Model file for the job. Use its own axes, mm. A direction names the side the tool comes from. Give positions to 0.01 mm unless a question says otherwise; leave off trailing zeros. Order: outer loops, then holes, each group sorted by start corner. A loop starts at its lowest first (then second) coordinate and runs counter-clockwise, first axis right, second up. Notation, with made-up numbers: (38, 7) - (92, 7) arc R8 cw to (92, 18) - close; hole circle Ø9 at (42, 70.5). An arc over 180 degrees is marked (long way). Use CSV: the item, a comma, the result in double quotes. Start each with the question number.
(1) Band-saw the part on A-A, the plane z = -0.7. Give the cut face in (x, y), then the cut area to 3 significant figures.
(2) Pull direction X, two halves, no side cores. Call faces 3 (the flat face through (15, -1, -1)), 4 (the cylindrical face through (-4.524, -1.065, -0.219)), 5 (the flat face through (-15, -1, 40.5)), 6 (the flat face through (-15, -1, -7)): +X half, -X half, draft (parallel to the pull), parting line (faces both ways), or undercut.
(3) Band-saw the part on B-B, the plane x = -6.05. Give the cut face in (y, z).
(4) Tool access for faces 1 (the flat face through (-30, -1, 27.65)), 2 (the cylindrical face through (7.452, -1.065, 13.019)): list every direction of +Z, -Z, +X, -X, +Y, -Y with a clear straight run to the whole face (end or side of a thin tool).
(5) Band-saw the part on C-C, the plane y = -0.95. Count the separate pieces of the cut face and the enclosed holes in it, then the cut area to 3 significant figures.
(6) Probe L1, parallel to Z at x = -42, y = -1.3 (3 decimals); L2, parallel to Z at x = 9, y = -1.2; L3, parallel to X at y = -1.55, z = 35.5. List the from-to ranges inside material, lowest first.
(7) Drop a flat-ended pin along its axis: pin 1 Ø1.9 at (x, z) = (6.05, -0.7) entering from -Y. Give the stop position or say it passes through.
(8) Band-saw the part on D-D, the plane z = 11.6. Give the cut face in (x, y).
from build123d import *

# Parameters (mm, degrees)
F0_W     = 30
F0_H     = 81
F1_DEPTH = 2.1
F2_R     = 2.1
F2_R_2   = 1.6
F3_DEPTH = 2.101
F4_W     = 2.1
F4_H     = 12.85
F5_DEPTH = 30
F6_R     = 1.1
F7_DEPTH = 25


with BuildPart() as f1:
    # F0 (on Front) → F1 (new body)
    with BuildSketch(Plane.XZ):
        Rectangle(F0_W, F0_H)
    extrude(amount=F1_DEPTH)

    # F2 (on face) → F3 (cut, through all)
    with BuildSketch(Plane.XZ.offset(2.1)):
        with Locations((9, 35.6)):
            Circle(F2_R)
        with Locations((9, 11.6)):
            Circle(F2_R)
        with Locations((-9, 35.6)):
            Circle(F2_R)
        with Locations((-9, 11.6)):
            Circle(F2_R)
        with Locations((9, -9.2)):
            Circle(F2_R)
        with Locations((-9, -9.2)):
            Circle(F2_R)
        with Locations((6.05, -0.7)):
            Circle(F2_R_2)
        with Locations((-6.05, -0.7)):
            Circle(F2_R_2)
    extrude(amount=-F3_DEPTH, mode=Mode.SUBTRACT)

    # F4 (on face) → F5 (join)
    with BuildSketch(Plane(origin=(-15, 0, 0), x_dir=(0, -1, 0), z_dir=(-1, 0, 0))):
        with Locations((1.05, 34.075)):
            Rectangle(F4_W, F4_H)
    extrude(amount=F5_DEPTH)

    # F6 (on face) → F7 (cut)
    with BuildSketch(Plane.XZ.offset(2.1)):
        with Locations((-42, 38.175)):
            Circle(F6_R)
        with Locations((-42, 29.975)):
            Circle(F6_R)
    extrude(amount=-F7_DEPTH, mode=Mode.SUBTRACT)


solid = f1.part
Answer block:
1,outline,"(-15, -2.1) - (-7.65, -2.1) - (-7.65, 0) - (-15, 0) - close; (-4.45, -2.1) - (4.45, -2.1) - (4.45, 0) - (-4.45, 0) - close; (7.65, -2.1) - (15, -2.1) - (15, 0) - (7.65, 0) - close"
1,area,"49.6 mm2"
2,face 3,"+X half"
2,face 4,"undercut"
2,face 5,"draft"
2,face 6,"-X half"
3,outline,"(-2.1, -40.5) - (0, -40.5) - (0, -2.3) - (-2.1, -2.3) - close; (-2.1, 0.9) - (0, 0.9) - (0, 40.5) - (-2.1, 40.5) - close"
4,face 1,"-Z, -X, +Y, -Y"
4,face 2,"+Y, -Y"
5,separate pieces,"1"
5,enclosed holes,"10"
5,area,"2,710 mm2"
6,L1,"z = 27.65 to 28.875, 31.075 to 37.075, 39.275 to 40.5"
6,L2,"z = -40.5 to -11.3, -7.1 to 9.5, 13.7 to 33.5, 37.7 to 40.5"
6,L3,"x = -45 to -11.1, -6.9 to 6.9, 11.1 to 15"
7,pin 1,"passes through"
8,outline,"(-15, -2.1) - (-11.1, -2.1) - (-11.1, 0) - (-15, 0) - close; (-6.9, -2.1) - (6.9, -2.1) - (6.9, 0) - (-6.9, 0) - close; (11.1, -2.1) - (15, -2.1) - (15, 0) - (11.1, 0) - close"
